```python
from build123d import *

# Parameters (mm, degrees)
SKETCH1_W           = 10
SKETCH1_H           = 5
SKETCH1_W_2         = 16
SKETCH1_H_2         = 4
BOSS_EXTRUDE1_DEPTH = 194.5
SKETCH2_W           = 6
SKETCH2_H           = 6
BOSS_EXTRUDE2_DEPTH = 20


with BuildPart() as part:
    # Sketch1 → Boss-Extrude1 (new body)
    with BuildSketch(Plane(origin=(0, 0, 0), x_dir=(0, 1, 0), z_dir=(0, 0, 1))):
        with Locations((0, -4.5)):
            Rectangle(SKETCH1_W, SKETCH1_H)
        Rectangle(SKETCH1_W_2, SKETCH1_H_2)
    extrude(amount=-BOSS_EXTRUDE1_DEPTH)

    # Sketch2 → Boss-Extrude2 (add)
    with BuildSketch(Plane(origin=(0, 0, -194.5), x_dir=(1, 0, 0), z_dir=(0, 0, -1))):
        with Locations((2.5, 0)):
            Rectangle(SKETCH2_W, SKETCH2_H)
    extrude(amount=BOSS_EXTRUDE2_DEPTH)


solid = part.part
```
Part model, mm, in its own coordinate system. A direction names the side the tool comes from. Round coordinates to 2 decimals unless told otherwise and drop trailing zeros. Loops run counter-clockwise (first coordinate to the right, second up) from the corner with the lowest first, then second, coordinate; pieces in that order, holes last.
1. Slice it at C-C (z = -197). Give the cut face in (x, y).
Solutions:
outline: (-0.5, -3) - (5.5, -3) - (5.5, 3) - (-0.5, 3) - close
2. Slice it at B-B (x = 3.5). Give the cut face in (y, z), and give its area (4 significant figures).
Solutions:
outline: (-5, -194.5) - (-3, -194.5) - (-3, -214.5) - (3, -214.5) - (3, -194.5) - (5, -194.5) - (5, 0) - (-5, 0) - close
area: 2,065 mm2
3. 3-axis set-ups, long thin cutter, end or side, ignore diameter. For faces 1 (the face through (2, 3, -204)), 2 (the face through (5.5, 0, -204)), 3 (the face through (5, -5, -96)), 4 (the face through (5, 5, -96)), 5 (the face through (-0.5, 0, -204)): which of +Z, -Z, +X, -X, +Y, -Y reach the whole face in a straight line?
Solutions:
face 1: -Z, +X, -X, +Y
face 2: -Z, +X, +Y, -Y
face 3: +Z, -Z, +X, -Y
face 4: +Z, -Z, +X, +Y
face 5: -Z, -X, +Y, -Y
4. Drill centre lines: line 1 along Y through (x, z) = (3, -134); line 2 along Z through (x, y) = (2.5, -4); line 3 along X through (y, z) = (-5.25, -55.5). Where is each one in solid material? Low to high.
Solutions:
line 1: y = -5 to 5
line 2: z = -194.5 to 0
line 3: x = -2 to 2
5. Flat gauge pins, fed straight in: pin 1 (1.5 mm diameter, centred on x = 5.5, z = -162.5, fed in from -Y); pin 2 (5 mm diameter, centred on x = 5, y = -6, fed in from +Z); pin 3 (6.5 mm diameter, centred on y = -0.5, z = -207.5, fed in from +X); pin 4 (2 mm diameter, centred on x = 5.5, y = 4.5, fed in from -Z). Where does each tip first touch, or does it go through?
Solutions:
pin 1: stops at y = -5
pin 2: stops at z = 0
pin 3: stops at x = 5.5
pin 4: stops at z = -194.5
6. Slice it at A-A (y = 0.25). Give the cut face in (x, z), and give its area (3 significant figures).
Solutions:
outline: (-2, -194.5) - (-0.5, -194.5) - (-0.5, -214.5) - (5.5, -214.5) - (5.5, -194.5) - (7, -194.5) - (7, 0) - (-2, 0) - close
area: 1,870 mm2
